Design review of the part built by this model. Coordinates are the model's own, in mm. Round coordinates to 2 decimals unless told otherwise and drop trailing zeros. Order: outer loops, then holes, each group sorted by start corner. A loop starts at its lowest first (then second) coordinate and runs counter-clockwise, first axis right, second up. Notation, with made-up numbers: (-30.5, 29.5) - (17.5, 29.5) arc R29 ccw to (17.5, 67.5) - close; hole circle Ø6 at (-20.5, 58). An arc over 180 degrees is marked (long way). Use CSV: the item, a comma, the result in double quotes. Start each with the question number.
from build123d import *

# Parameters (mm, degrees)
F0_R     = 37.476533
F1_DEPTH = 196.006492
F2_W     = 109.178945
F2_H     = 81.75566
F3_DEPTH = 113.557346


with BuildPart() as f1:
    # F0 (on Front) → F1 (new body)
    with BuildSketch(Plane.XZ):
        with Locations((36.363707, 23.673844)):
            Circle(F0_R)
    extrude(amount=F1_DEPTH)


with BuildPart() as f3:
    # F2 (on Top) → F3 (new body)
    with BuildSketch(Plane.XY):
        with Locations((17.131656, -108.327765)):
            Rectangle(F2_W, F2_H)
    extrude(amount=F3_DEPTH)

    # F4: intersect F1
    add(f1.part, mode=Mode.INTERSECT)


solid = f3.part
Q1. Clearance check with flat-ended pins moving along their axes: pin 1 (1.5 mm diameter, centred on y = -138, z = 39, fed in from -X); pin 2 (6 mm diameter, centred on y = -110, z = 11.5, fed in from -X); pin 3 (3 mm diameter, centred on y = -86, z = 27, fed in from -X). State where each tip first meets the part, or that it passes through.
Q2. Take a section at A-A (y = -77). State the section outline as (x, z) points.
Q3. For L1, parallel to X at y = -84.5, z = 39; L2, parallel to Z at x = 32, y = -111.5; L3, parallel to Z at x = 16.5, y = -74, list the stretches that pass through material, from the lowest coordinate up. Write a range as [from, to].
Q4. Take a section at B-B (x = 16.5). State the section outline as (y, z) points, plus the area to 3 significant figures.
Findings below:
1,pin 1,"stops at x = 1.84"
1,pin 2,"stops at x = 0.03"
1,pin 3,"stops at x = -1.07"
2,outline,"(7.31, 0) - (65.42, 0) arc R37.48 ccw to (71.72, 11.25) - (71.72, 36.1) arc R37.48 ccw (long way) to start"
3,L1,"x = [2.16, 70.56]"
3,L2,"z = [0, 60.9]"
3,L3,"z = [0, 55.45]"
4,outline,"(-149.21, 0) - (-67.45, 0) - (-67.45, 55.45) - (-149.21, 55.45) - close"
4,area,"4,530 mm^2"
